from build123d import *

# Parameters (mm, degrees)
BOSS_EXTRUDE1_DEPTH     = 39.35
CUT_EXTRUDE2_DEPTH      = 33.73
CUT_EXTRUDE2_DEPTH_BACK = 3
SKETCH3_R               = 5.15
CUT_EXTRUDE3_DEPTH      = 33.73
CUT_EXTRUDE4_DEPTH      = 87.647311883
CUT_EXTRUDE4_DEPTH_BACK = 87.647311883
SKETCH3_5_R             = 3.1
SKETCH3_5_R_2           = 10.1
SKETCH3_5_R_3           = 1.6
SKETCH3_5_W             = 20.675
SKETCH3_5_H             = 20.2
SKETCH3_5_W_2           = 5.027537917
SKETCH3_5_H_2           = 3.2
SKETCH3_5_W_3           = 5.03
SKETCH3_6_R             = 1.6
CUT_EXTRUDE5_DEPTH      = 87.647311883
BOSS_EXTRUDE2_DEPTH     = 4
BOSS_EXTRUDE3_DEPTH     = 4
CUT_EXTRUDE6_DEPTH      = 92.909209967
CUT_EXTRUDE6_DEPTH_BACK = 92.909209967
CUT_EXTRUDE7_DEPTH      = 2.5
SKETCH10_W              = 47.35
SKETCH10_H              = 38.73
BOSS_EXTRUDE5_DEPTH     = 4
CHAMFER3_SIZE           = 16
CHAMFER3_SIZE_2         = 27.712812921


with BuildPart() as part:
    # Sketch1 → Boss-Extrude1 (new body)
    with BuildSketch(Plane.XY):
        Polygon((-68.943174111, 38.106680783), (-32.943174111, 38.106680783), (-32.943174111, 3.376680783), (8.406825889, 3.376680783), (8.406825889, -0.623319217), (-68.943174111, -0.623319217), (-68.943174111, 3.376680783), (-36.943174111, 3.376680783), (-36.943174111, 34.106680783), (-68.943174111, 34.106680783), align=None)
    extrude(amount=BOSS_EXTRUDE1_DEPTH)

    # Sketch3 → Cut-Extrude2 (cut, two sides: drawn at the far end of the back side and taken through both)
    with BuildSketch(Plane(origin=(0, 3.376680783, 0), x_dir=(1, 0, 0), z_dir=(0, 1, 0)).offset(-CUT_EXTRUDE2_DEPTH_BACK)):
        with Locations(Location((-52.943174111, -19.675, 0), (0, 0, 90))):
            Circle(SKETCH3_R)
    extrude(amount=CUT_EXTRUDE2_DEPTH + CUT_EXTRUDE2_DEPTH_BACK, mode=Mode.SUBTRACT)

    # Sketch3<4> → Cut-Extrude3 (cut)
    with BuildSketch(Plane(origin=(0, 3.376680783, 0), x_dir=(1, 0, 0), z_dir=(0, 1, 0))):
        with BuildLine():
            Line((-47.611429556, -21.025), (-45.3116605, -21.025))
            Line((-45.3116605, -21.025), (-45.3116605, -18.325))
            Line((-45.3116605, -18.325), (-47.611429556, -18.325))
            ThreePointArc((-47.611429556, -18.325), (-47.485400066, -18.994777629), (-47.443174111, -19.675))
            ThreePointArc((-47.443174111, -19.675), (-47.485400066, -20.355222371), (-47.611429556, -21.025))
        make_face()
        with BuildLine():
            Line((-60.574687722, -18.325), (-60.574687722, -21.025))
            Line((-60.574687722, -21.025), (-58.274918666, -21.025))
            ThreePointArc((-58.274918666, -21.025), (-58.443174111, -19.675), (-58.274918666, -18.325))
            Line((-58.274918666, -18.325), (-60.574687722, -18.325))
        make_face()
    extrude(amount=CUT_EXTRUDE3_DEPTH, mode=Mode.SUBTRACT)

    # Sketch3<5> → Cut-Extrude4 (cut, two sides: drawn at the far end of the back side and taken through both)
    with BuildSketch(Plane(origin=(0, 3.376680783, 0), x_dir=(1, 0, 0), z_dir=(0, 1, 0)).offset(-CUT_EXTRUDE4_DEPTH_BACK)):
        with Locations(Location((-52.943174111, -19.675, 0), (0, 0, 270))):
            Circle(SKETCH3_5_R)
        with Locations((-12.268174111, -19.675)):
            Circle(SKETCH3_5_R_2)
        with Locations((-4.768174111, -32.665381057)):
            Circle(SKETCH3_5_R_3)
        with Locations((-4.768174111, -6.684618943)):
            Circle(SKETCH3_5_R_3)
        with Locations((-27.268174111, -19.675)):
            Circle(SKETCH3_5_R_3)
        with Locations((0.261825889, -32.665381057)):
            Circle(SKETCH3_5_R_3)
        with Locations((0.261825889, -6.684618943)):
            Circle(SKETCH3_5_R_3)
        with Locations((-1.930674111, -19.675)):
            Rectangle(SKETCH3_5_W, SKETCH3_5_H)
        with Locations((-24.754405152, -19.675)):
            Rectangle(SKETCH3_5_W_2, SKETCH3_5_H_2)
        with Locations((-2.253174111, -32.665381057)):
            Rectangle(SKETCH3_5_W_3, SKETCH3_5_H_2)
        with Locations((-2.253174111, -6.684618943)):
            Rectangle(SKETCH3_5_W_3, SKETCH3_5_H_2)
    extrude(amount=CUT_EXTRUDE4_DEPTH + CUT_EXTRUDE4_DEPTH_BACK, mode=Mode.SUBTRACT)

    # Sketch3<6> → Cut-Extrude5 (cut, through all)
    with BuildSketch(Plane(origin=(0, 3.376680783, 0), x_dir=(1, 0, 0), z_dir=(0, 1, 0))):
        with Locations(Location((-52.943174111, -34.675, 0), (0, 0, 180))):
            Circle(SKETCH3_6_R)
        with Locations(Location((-65.933555168, -27.175, 0), (0, 0, 180))):
            Circle(SKETCH3_6_R)
        with Locations(Location((-65.933555168, -12.175, 0), (0, 0, 180))):
            Circle(SKETCH3_6_R)
        with Locations(Location((-52.943174111, -4.675, 0), (0, 0, 180))):
            Circle(SKETCH3_6_R)
        with Locations(Location((-39.952793054, -12.175, 0), (0, 0, 180))):
            Circle(SKETCH3_6_R)
        with Locations(Location((-39.952793054, -27.175, 0), (0, 0, 180))):
            Circle(SKETCH3_6_R)
    extrude(amount=CUT_EXTRUDE5_DEPTH, mode=Mode.SUBTRACT)

    # Sketch4 → Boss-Extrude2 (add)
    with BuildSketch(Plane.XY.offset(39.35)):
        Polygon((-68.943174111, 38.106680783), (-68.943174111, 34.106680783), (-36.943174111, 34.106680783), (-36.943174111, 3.376680783), (-68.943174111, 3.376680783), (-68.943174111, -0.623319217), (8.406825889, -0.623319217), (8.406825889, 38.106680783), align=None)
    extrude(amount=BOSS_EXTRUDE2_DEPTH)

    # Sketch5 → Boss-Extrude3 (add)
    with BuildSketch(Plane(origin=(0, 0, 0), x_dir=(-1, 0, 0), z_dir=(0, 0, -1))):
        Polygon((68.943174111, 38.106680783), (68.943174111, 34.106680783), (36.943174111, 34.106680783), (36.943174111, 3.376680783), (68.943174111, 3.376680783), (68.943174111, -0.623319217), (-8.406825889, -0.623319217), (-8.406825889, 38.106680783), align=None)
    extrude(amount=BOSS_EXTRUDE3_DEPTH)

    # Sketch6 → Cut-Extrude6 (cut, two sides: drawn at the far end of the back side and taken through both)
    with BuildSketch(Plane.XY.offset(43.35).offset(-CUT_EXTRUDE6_DEPTH_BACK)):
        Polygon((-32.943174111, 38.106680783), (5.861825889, 3.376680783), (5.861825889, -0.623319217), (8.406825889, -0.623319217), (8.406825889, 38.106680783), align=None)
    extrude(amount=CUT_EXTRUDE6_DEPTH + CUT_EXTRUDE6_DEPTH_BACK, mode=Mode.SUBTRACT)

    # Sketch8 → Cut-Extrude7 (cut)
    with BuildSketch(Plane.XZ.offset(-34.106680783)):
        Polygon((-65.933555168, 15.408161507), (-68.733555168, 13.791580754), (-68.733555168, 10.558419246), (-65.933555168, 8.941838493), (-63.133555168, 10.558419246), (-63.133555168, 13.791580754), align=None)
        Polygon((-65.933555168, 30.408161507), (-68.733555168, 28.791580754), (-68.733555168, 25.558419246), (-65.933555168, 23.941838493), (-63.133555168, 25.558419246), (-63.133555168, 28.791580754), align=None)
        Polygon((-52.943174111, 1.441838493), (-50.143174111, 3.058419246), (-50.143174111, 6.291580754), (-52.943174111, 7.908161507), (-55.743174111, 6.291580754), (-55.743174111, 3.058419246), align=None)
        Polygon((-39.952793054, 8.941838493), (-37.152793054, 10.558419246), (-37.152793054, 13.791580754), (-39.952793054, 15.408161507), (-42.752793054, 13.791580754), (-42.752793054, 10.558419246), align=None)
        Polygon((-39.952793054, 23.941838493), (-37.152793054, 25.558419246), (-37.152793054, 28.791580754), (-39.952793054, 30.408161507), (-42.752793054, 28.791580754), (-42.752793054, 25.558419246), align=None)
        Polygon((-52.943174111, 37.908161507), (-55.743174111, 36.291580754), (-55.743174111, 33.058419246), (-52.943174111, 31.441838493), (-50.143174111, 33.058419246), (-50.143174111, 36.291580754), align=None)
    extrude(amount=-CUT_EXTRUDE7_DEPTH, mode=Mode.SUBTRACT)

    # Sketch10 → Boss-Extrude5 (add)
    with BuildSketch(Plane.ZY.offset(68.943174111)):
        with Locations((19.675, 18.741680783)):
            Rectangle(SKETCH10_W, SKETCH10_H)
    extrude(amount=BOSS_EXTRUDE5_DEPTH)

    # Chamfer3
    # the kernel refuses this chamfer: 27.712812921, 16 mm, written as the material it takes off along each edge
    with BuildSketch(Plane(origin=(-72.943174111, -72.318742746, -4), x_dir=(-0.05789386240267147, 0, 0.9983227437537926), z_dir=(0, 1, 0))) as chamfer3_piece_1:
        Polygon((CHAMFER3_SIZE * 0.998322743754, CHAMFER3_SIZE * 0.0578938624027), (-CHAMFER3_SIZE_2 * 0.0578938624029, CHAMFER3_SIZE_2 * 0.998322743757), (0, 0), align=None)
    extrude(amount=182.120847059, mode=Mode.SUBTRACT)
    with BuildSketch(Plane(origin=(-72.943174111, 109.802104312, 43.35), x_dir=(0.9998132206222079, 0, 0.019326765612700702), z_dir=(0, -1, 0))) as chamfer3_piece_2:
        Polygon((CHAMFER3_SIZE_2 * 0.999813220626, -CHAMFER3_SIZE_2 * 0.0193267656128), (-CHAMFER3_SIZE * 0.0193267656127, -CHAMFER3_SIZE * 0.999813220622), (0, 0), align=None)
    extrude(amount=182.120847059, mode=Mode.SUBTRACT)


solid = part.part
Could you check a few things on this model? Use its own coordinates, in mm. A direction names the side the tool comes from. Coordinates: 2 decimals unless noted, no trailing zeros. Order: outer loops, then holes, each group sorted by start corner. A loop starts at its lowest first (then second) coordinate and runs counter-clockwise, first axis right, second up.
Q1. Suppose I cut it at C-C on y = 21.5. Please give me the cut outline in (x, z), and give its area (3 significant figures).
Q2. Thinking about a two-plate mould opening in Z: for faces 1 (the flat face through (-13.812, 20.985, -2.028)), 2 (the flat face through (-51, 37.107, 17)), which applies, released by +Z, released by -Z, zero draft, split by the parting line, or undercut?
Q3. Will these pins go through, and if not, where does the flat tip stop? pin 1 (1.9 mm diameter, centred on x = -52.94, z = 34.67, fed in from +Y); pin 2 (6 mm diameter, centred on y = 11.5, z = 26.5, fed in from +X); pin 3 (6 mm diameter, centred on x = -52.94, z = 19.68, fed in from +Y).
Q4. Suppose I cut it at D-D on y = 35.5. Give the number of separate pieces and of enclosed holes in the cut face, and give its area (3 significant figures).
Q5. Which directions (+Z, -Z, +X, -X, +Y, -Y) give clear straight access to the entire face, cutting with the end or side of a thin tool? Please do faces 3 (the flat face through (-22, 3.377, 24)), 4 (the flat face through (-2, 1, 34.265)), 5 (the flat face through (-51.56, 35.34, 32.24)), 6 (the flat face through (-3, 1, 9.575)).
Q6. Suppose I cut it at B-B on x = -1. Please give me the cut outline in (y, z) (3 decimals), and give its area (3 significant figures).
Q7. Suppose I cut it at A-A on y = 13. Please give me the cut outline in (x, z), and give its area (3 significant figures).
Q8. Please list where these lines run through material, in increasing order: L1, parallel to X at y = 8, z = 23; L2, parallel to Y at x = -50, z = 32; L3, parallel to Z at x = -24.5, y = 27.5.
Answer:
1. outline: (-72.94, 12) - (-68.94, 9.69) - (-68.94, 29.66) - (-72.94, 27.35) - close; (-36.94, -4) - (-14.39, -4) - (-14.39, 0) - (-32.94, 0) - (-32.94, 39.35) - (-14.39, 39.35) - (-14.39, 43.35) - (-36.94, 43.35) - close
1. area: 408 mm2
2. face 1: zero draft
2. face 2: undercut
3. pin 1: stops at y = 3.38
3. pin 2: stops at x = -32.94
3. pin 3: passes through
4. separate pieces: 1
4. enclosed holes: 9
4. area: 1,220 mm2
5. face 3: +X, +Y
5. face 4: +Y, -Y
5. face 5: none
5. face 6: +X, +Y, -Y
6. outline: (-0.623, -4) - (9.518, -4) - (9.518, 0) - (3.377, 0) - (3.377, 5.085) - (-0.623, 5.085) - close; (-0.623, 8.285) - (3.377, 8.285) - (3.377, 9.575) - (-0.623, 9.575) - close; (-0.623, 29.775) - (3.377, 29.775) - (3.377, 31.065) - (-0.623, 31.065) - close; (-0.623, 34.265) - (3.377, 34.265) - (3.377, 39.35) - (9.518, 39.35) - (9.518, 43.35) - (-0.623, 43.35) - close
6. area: 132 mm2
7. outline: (-72.94, 12) - (-68.94, 9.69) - (-68.94, 29.66) - (-72.94, 27.35) - close; (-36.94, -4) - (-4.89, -4) - (-4.89, 0) - (-32.94, 0) - (-32.94, 39.35) - (-4.89, 39.35) - (-4.89, 43.35) - (-36.94, 43.35) - close
7. area: 484 mm2
8. L1: x = -72.94 to -68.94, -36.94 to -32.94
8. L2: y = -0.62 to 3.38, 34.11 to 38.11
8. L3: z = -4 to 0, 39.35 to 43.35
